Can you work these out from the model? Positions are in its coordinate system, mm. Face numbers are marked on the shaded views. A direction names the side the tool comes from. Coordinates: 2 decimals unless noted, no trailing zeros. Order: outer loops, then holes, each group sorted by start corner. A loop starts at its lowest first (then second) coordinate and runs counter-clockwise, first axis right, second up. Notation, with made-up numbers: (76, -12) - (93, -12) arc R36 ccw to (93, 25) - close; hole circle Ø2 at (9, 4). An arc over 180 degrees is marked (long way). Return JSON: item names as keys, results as strings. Group by question number.
1) For pin 1 Ø3 at (x, z) = (4.5, -3) entering from -Y; pin 2 Ø1.8 at (x, z) = (4.7, 28) entering from -Y; pin 3 Ø8 at (x, y) = (19, 7.5) entering from +Z; pin 4 Ø19.5 at (x, z) = (20.85, 11.85) entering from -Y, each with a flat end and sliding along its axis, tell me the tip position at first contact or that it passes through.
2) If we mould it in two halves opening along Y, with no side actions, what happens to the marked faces 4, 5 and 6? For each: pulls with the +Y half, pulls with the -Y half, needs draft (parallel to the pull), parting line crosses it, or undercut.
3) Which directions (+Z, -Z, +X, -X, +Y, -Y) give clear straight access to the entire face, cutting with the end or side of a thin tool? Please do the marked faces 1, 2 and 3.
4) Imagine slicing it at C-C (z = 11.85). Write out the boundary of the cut face in (x, y), and give its area (3 significant figures).
5) Imagine slicing it at B-B (z = -4.3). Write out the boundary of the cut face in (x, y), and give its area (3 significant figures).
6) Imagine slicing it at D-D (x = 37). Write out the boundary of the cut face in (y, z), and give its area (3 significant figures).
7) If I drill on line 1 along X through (y, z) = (13.6, 28); line 2 along X through (y, z) = (12.25, -4.3); line 3 along X through (y, z) = (11, -4.3), over which ranges is the centre line in solid material (lowest first)?
8) Imagine slicing it at A-A (y = 8). Write out the boundary of the cut face in (x, z), and give its area (3 significant figures).
```python
from build123d import *

# Parameters (mm, degrees)
SKETCH1_W           = 42
SKETCH1_H           = 9
BOSS_EXTRUDE1_DEPTH = 12
SKETCH2_W           = 42
SKETCH2_H           = 42
BOSS_EXTRUDE2_DEPTH = 4
FILLET1_R           = 2.5
FILLET2_R           = 2.5
FILLET3_R           = 2.5
FILLET4_R           = 2.5
FILLET5_R           = 2.5
FILLET6_R           = 2.5
SKETCH3_R           = 7.5
SKETCH3_R_2         = 1.5
SKETCH3_R_3         = 1.342252065
CUT_EXTRUDE1_DEPTH  = 20
SKETCH4_R           = 3
CUT_EXTRUDE2_DEPTH  = 5
SKETCH5_R           = 4
CUT_EXTRUDE3_DEPTH  = 9


with BuildPart() as part:
    # Sketch1 → Boss-Extrude1 (new body)
    with BuildSketch(Plane(origin=(0, 0, 0), x_dir=(1, 0, 0), z_dir=(0, 1, 0))):
        with Locations((21, 4.5)):
            Rectangle(SKETCH1_W, SKETCH1_H)
    extrude(amount=BOSS_EXTRUDE1_DEPTH)

    # Sketch2 → Boss-Extrude2 (add)
    with BuildSketch(Plane(origin=(0, 12, 0), x_dir=(1, 0, 0), z_dir=(0, 1, 0))):
        with Locations((21, -12)):
            Rectangle(SKETCH2_W, SKETCH2_H)
    extrude(amount=BOSS_EXTRUDE2_DEPTH)

    # Fillet1
    fillet1_edges = [part.edges().sort_by_distance(p)[0] for p in [
        (0, 14, 33),
    ]]
    fillet(fillet1_edges, radius=FILLET1_R)

    # Fillet2
    fillet2_edges = [part.edges().sort_by_distance(p)[0] for p in [
        (0, 8, -9),
    ]]
    fillet(fillet2_edges, radius=FILLET2_R)

    # Fillet3
    fillet3_edges = [part.edges().sort_by_distance(p)[0] for p in [
        (0, 6, 0),
    ]]
    fillet(fillet3_edges, radius=FILLET3_R)

    # Fillet4
    fillet4_edges = [part.edges().sort_by_distance(p)[0] for p in [
        (42, 14, 33),
    ]]
    fillet(fillet4_edges, radius=FILLET4_R)

    # Fillet5
    fillet5_edges = [part.edges().sort_by_distance(p)[0] for p in [
        (42, 6, 0),
    ]]
    fillet(fillet5_edges, radius=FILLET5_R)

    # Fillet6
    fillet6_edges = [part.edges().sort_by_distance(p)[0] for p in [
        (42, 8, -9),
    ]]
    fillet(fillet6_edges, radius=FILLET6_R)

    # Sketch3 → Cut-Extrude1 (cut)
    with BuildSketch(Plane(origin=(0, 16, 0), x_dir=(1, 0, 0), z_dir=(0, 1, 0))):
        with Locations(Location((20.85, -11.85, 0), (0, 0, 270))):
            Circle(SKETCH3_R)
        with Locations(Location((4.7, -28, 0), (0, 0, 270))):
            Circle(SKETCH3_R_2)
        with Locations(Location((37, -28, 0), (0, 0, 270))):
            Circle(SKETCH3_R_2)
        with Locations(Location((37, 4.3, 0), (0, 0, 270))):
            Circle(SKETCH3_R_2)
        with Locations(Location((4.7, 4.3, 0), (0, 0, 270))):
            Circle(SKETCH3_R_3)
    extrude(amount=-CUT_EXTRUDE1_DEPTH, mode=Mode.SUBTRACT)

    # Sketch4 → Cut-Extrude2 (cut)
    with BuildSketch(Plane.XZ):
        with Locations(Location((4.7, -4.3, 0), (0, 0, 270))):
            Circle(SKETCH4_R)
        with Locations(Location((37, -4.3, 0), (0, 0, 270))):
            Circle(SKETCH4_R)
    extrude(amount=-CUT_EXTRUDE2_DEPTH, mode=Mode.SUBTRACT)

    # Sketch5 → Cut-Extrude3 (cut)
    with BuildSketch(Plane(origin=(0, 0, -9), x_dir=(-1, 0, 0), z_dir=(0, 0, -1))):
        with Locations((-27, 8)):
            Circle(SKETCH5_R)
    extrude(amount=-CUT_EXTRUDE3_DEPTH, mode=Mode.SUBTRACT)


solid = part.part
```
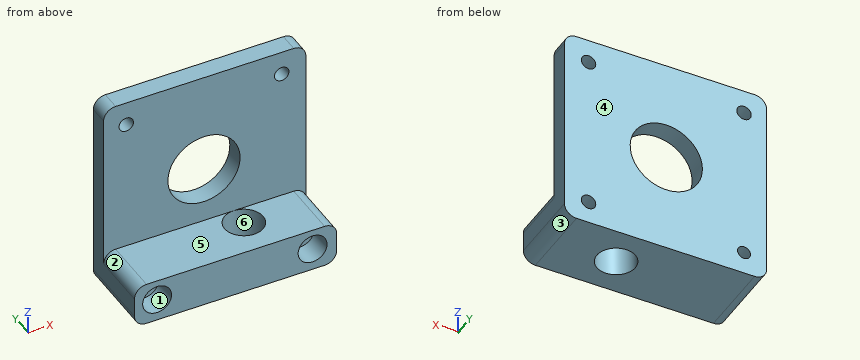
Calculated:
{
 "1": {"pin 1": "y = 5", "pin 2": "through", "pin 3": "z = 0", "pin 4": "y = 12"},
 "2": {"face 4": "pulls with the +Y half", "face 5": "needs draft", "face 6": "undercut"},
 "3": {"face 1": "-Y", "face 2": "+Z, -X, -Y", "face 3": "-Z, +X, +Y, -Y"},
 "4": {"outline": "(0, 12) - (13.35, 12) - (13.35, 16) - (0, 16) - close; (28.35, 12) - (42, 12) - (42, 16) - (28.35, 16) - close", "area": "108 mm2"},
 "5": {"outline": "(0, 0) - (1.7, 0) - (1.7, 5) - (3.36, 5) - (3.36, 16) - (0, 16) - close; (6.04, 5) - (7.7, 5) - (7.7, 0) - (34, 0) - (34, 5) - (35.5, 5) - (35.5, 16) - (6.04, 16) - close; (38.5, 5) - (40, 5) - (40, 0) - (42, 0) - (42, 16) - (38.5, 16) - close; hole circle Ø8 at (27, 8)", "area": "499 mm2"},
 "6": {"outline": "(0, -9) - (16, -9) - (16, -5.8) - (5, -5.8) - (5, -7.3) - (0, -7.3) - close; (0, -1.3) - (5, -1.3) - (5, -2.8) - (16, -2.8) - (16, 26.5) - (12, 26.5) - (12, 0) - (0, 0) - close; (12, 29.5) - (16, 29.5) - (16, 33) - (12, 33) - close", "area": "201 mm2"},
 "7": {"line 1": "0 to 3.2, 6.2 to 35.5, 38.5 to 42", "line 2": "0 to 3.36, 6.04 to 35.5, 38.5 to 42", "line 3": "0 to 3.36, 6.04 to 24.35, 29.65 to 35.5, 38.5 to 42"},
 "8": {"outline": "(0, -6.5) arc R2.5 ccw to (2.5, -9) - (23, -9) - (23, 0) - (2.5, 0) arc R2.5 ccw to (0, -2.5) - close; (31, -9) - (39.5, -9) arc R2.5 ccw to (42, -6.5) - (42, -2.5) arc R2.5 ccw to (39.5, 0) - (31, 0) - close; hole circle Ø2.68 at (4.7, -4.3); hole circle Ø3 at (37, -4.3)", "area": "288 mm2"}
}
